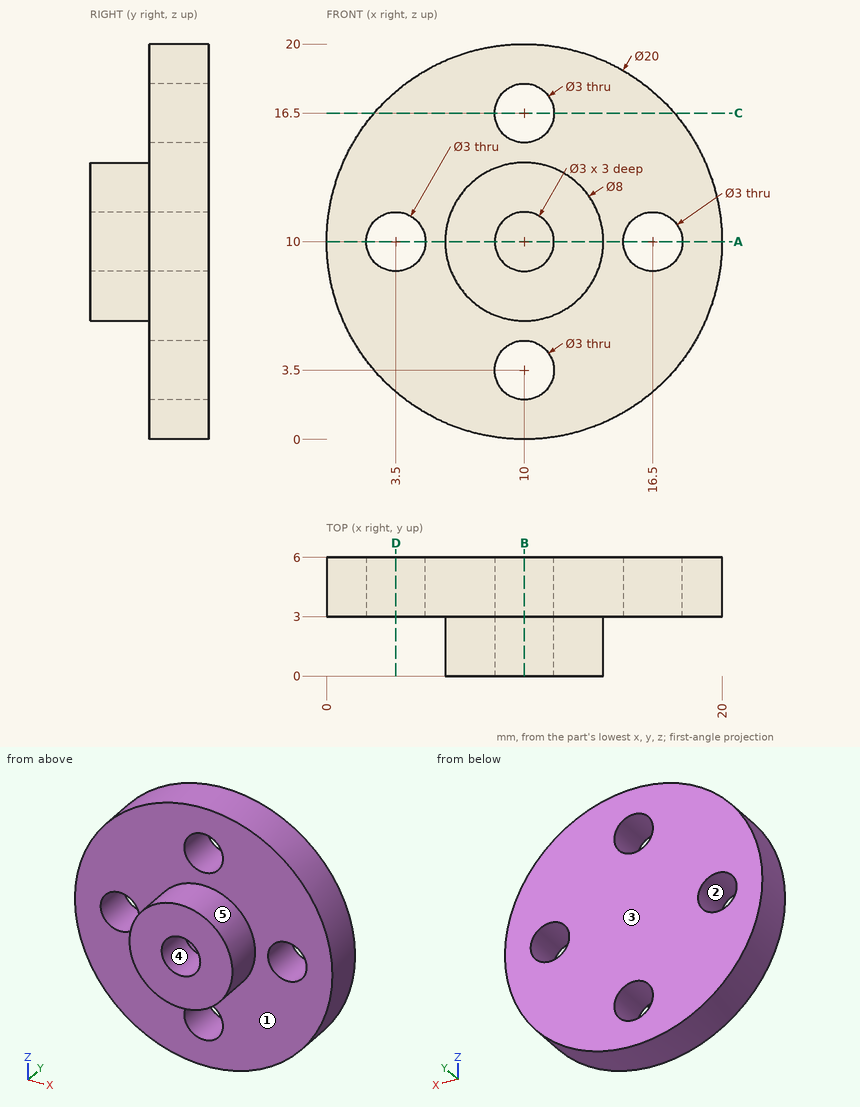
Geometry check sheet. Reference: drawing and pictorial views, mm from the part's lowest x, y, z. A direction names the side the tool comes from. Give positions to 0.01 mm unless a question says otherwise; leave off trailing zeros. Loops run counter-clockwise (first coordinate to the right, second up) from the corner with the lowest first, then second, coordinate; pieces in that order, holes last.
1. Set-up check for the marked faces 1 and 2: record each of +Z, -Z, +X, -X, +Y, -Y from which the full face is reachable in a straight line by a thin tool's end or side.
2. Section check A-A, the plane z = 10. Enter the section's corners in (x, y).
3. Mould release check, pull along Z, two halves, no side actions. Record for the marked faces 3, 4 and 5: released by +Z, released by -Z, zero draft, split by the parting line, or undercut.
4. Section check D-D, the plane x = 3.5. Enter the section's corners in (y, z), then the cut area to 3 significant figures.
5. Thickness scan on line 1 (X direction, y = 3.75, z = 10); line 2 (Z direction, x = 11.25, y = 4.15). Record the ranges inside material, lowest first.
6. Go/stop test with flat-tipped pins: pin 1 Ø3.5 at (x, z) = (3.5, 10) entering from -Y; pin 2 Ø1 at (x, y) = (11, 4.5) entering from -Z. Record where each tip stops, or that it passes through.
7. Section check B-B, the plane x = 10. Enter the section's corners in (y, z), then the cut area to 3 significant figures.
8. Section check C-C, the plane z = 16.5. Enter the section's corners in (x, y), then the cut area to 3 significant figures.
Geometry says:
1. face 1: -Y
1. face 2: +Y, -Y
2. outline: (0, 3) - (2, 3) - (2, 6) - (0, 6) - close; (5, 3) - (6, 3) - (6, 0) - (8.5, 0) - (8.5, 3) - (11.5, 3) - (11.5, 0) - (14, 0) - (14, 3) - (15, 3) - (15, 6) - (5, 6) - close; (18, 3) - (20, 3) - (20, 6) - (18, 6) - close
3. face 3: zero draft
3. face 4: undercut
3. face 5: split by the parting line
4. outline: (3, 2.4) - (6, 2.4) - (6, 8.5) - (3, 8.5) - close; (3, 11.5) - (6, 11.5) - (6, 17.6) - (3, 17.6) - close
4. area: 36.6 mm2
5. line 1: x = 0 to 2, 5 to 15, 18 to 20
5. line 2: z = 0.08 to 2.67, 4.33 to 15.67, 17.33 to 19.92
6. pin 1: stops at y = 3
6. pin 2: stops at z = 0.01
7. outline: (0, 6) - (3, 6) - (3, 5) - (6, 5) - (6, 15) - (3, 15) - (3, 14) - (0, 14) - (0, 11.5) - (3, 11.5) - (3, 8.5) - (0, 8.5) - close; (3, 0) - (6, 0) - (6, 2) - (3, 2) - close; (3, 18) - (6, 18) - (6, 20) - (3, 20) - close
7. area: 57.0 mm2
8. outline: (2.4, 3) - (8.5, 3) - (8.5, 6) - (2.4, 6) - close; (11.5, 3) - (17.6, 3) - (17.6, 6) - (11.5, 6) - close
8. area: 36.6 mm2
